Job drawing, mm, ordinate dimensions from the low corner. One solid piece. A direction names the side the tool comes from. Round coordinates to 2 decimals unless told otherwise and drop trailing zeros. Order: outer loops, then holes, each group sorted by start corner. A loop starts at its lowest first (then second) coordinate and runs counter-clockwise, first axis right, second up. Notation, with made-up numbers: (29, -29.5) -> (47, -29.5) arc R27 ccw to (47, -13.5) -> close; hole circle Ø8 at (38.25, -28.75). An arc over 180 degrees is marked (long way). Return JSON: item names as keys, results as strings. Group by question number.
Q1. Cut at D-D (x = 10). Write the cut outline in (y, z).
Q2. Flat gauge pins, fed straight in: pin 1 (1.1 mm diameter, centred on x = 41, z = 18, fed in from -Y); pin 2 (1.8 mm diameter, centred on x = 44.5, z = 13.5, fed in from -Y); pin 3 (0.9 mm diameter, centred on y = 2, z = 21.5, fed in from +X). Where does each tip first touch, or does it go through?
Q3. Mould opens along Z. For the marked faces 4, 5 and 6 say: +Z half, -Z half, draft (parallel to the pull), parting line (faces both ways), or undercut.
Q4. Cut at B-B (y = 5.25). Write the cut outline in (x, z).
Q5. Which spindle directions (+Z, -Z, +X, -X, +Y, -Y) get a long thin tool onto all of the face, cutting with end or side? Do the marked faces 1, 2 and 3. Say none if no direction does.
Q6. Probe line 1 along Z through (x, y) = (22, 2.75); line 2 along X through (y, z) = (8.75, 24.75) (1 decimal); line 3 along X through (y, z) = (2.5, 24) (1 decimal). List the from-to ranges inside material, lowest first.
Q7. Cut at A-A (x = 34). Write the cut outline in (y, z).
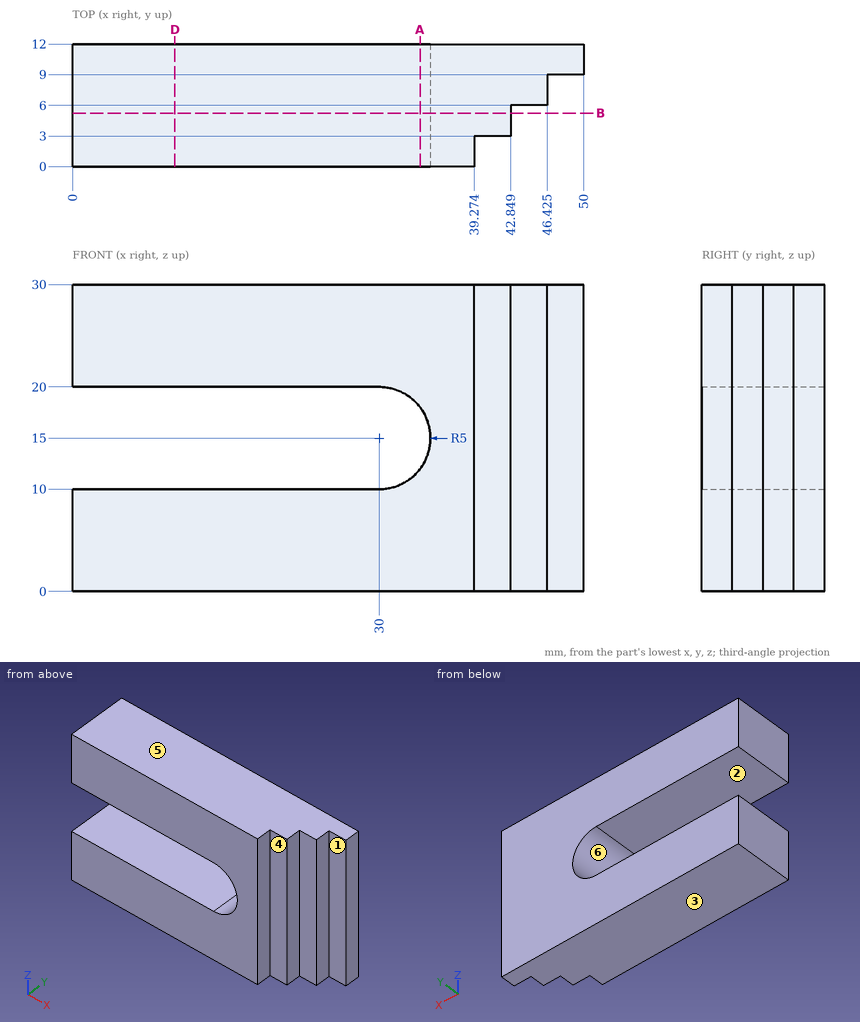
Solution:
{
 "1": {"outline": "(0, 0) -> (12, 0) -> (12, 10) -> (0, 10) -> close; (0, 20) -> (12, 20) -> (12, 30) -> (0, 30) -> close"},
 "2": {"pin 1": "stops at y = 3", "pin 2": "stops at y = 6", "pin 3": "stops at x = 39.27"},
 "3": {"face 4": "draft", "face 5": "+Z half", "face 6": "undercut"},
 "4": {"outline": "(0, 0) -> (42.85, 0) -> (42.85, 30) -> (0, 30) -> (0, 20) -> (30, 20) arc R5 cw to (30, 10) -> (0, 10) -> close"},
 "5": {"face 1": "+Z, -Z, +X, -Y", "face 2": "-X, +Y, -Y", "face 3": "-Z, +X, -X, +Y, -Y"},
 "6": {"line 1": "z = 0 to 10, 20 to 30", "line 2": "x = 0 to 46.4", "line 3": "x = 0 to 39.3"},
 "7": {"outline": "(0, 0) -> (12, 0) -> (12, 12) -> (0, 12) -> close; (0, 18) -> (12, 18) -> (12, 30) -> (0, 30) -> close"}
}
